Can you work these out from the model? Positions are in its coordinate system, mm. Face numbers are marked on the shaded views. A direction names the side the tool comes from. Round coordinates to 2 decimals unless told otherwise and drop trailing zeros. Loops run counter-clockwise (first coordinate to the right, second up) from the corner with the lowest first, then second, coordinate; pieces in that order, holes last. Notation, with made-up numbers: (7.25, 77.25) -> (55.25, 77.25) arc R35 ccw to (55.25, 116.25) -> close; hole circle Ø2 at (29, 16.5). An arc over 180 degrees is marked (long way). Write item = value, one per line.
from build123d import *

# Parameters (mm, degrees)
SKETCH1_W           = 86
SKETCH1_H           = 79
BOSS_EXTRUDE1_DEPTH = 36.5
CUT_EXTRUDE4_DEPTH  = 113.8543313
CUT_EXTRUDE6_DEPTH  = 117.39336237
SKETCH23_W          = 52.496433732
SKETCH23_H          = 95.180046085
CUT_EXTRUDE9_DEPTH  = 99.910462918
SKETCH26_W          = 80.038892534
SKETCH26_H          = 43.235962509
CUT_EXTRUDE10_DEPTH = 122.988754281
SKETCH27_R          = 10
BOSS_EXTRUDE2_DEPTH = 20
SKETCH28_R          = 9.1
CUT_EXTRUDE11_DEPTH = 20


with BuildPart() as part:
    # Sketch1 → Boss-Extrude1 (new body)
    with BuildSketch(Plane(origin=(0, 0, 0), x_dir=(1, 0, 0), z_dir=(0, 1, 0))):
        Polygon((-79.5, 16), (-79.5, -16), (-43, -39.5), (-43, 39.5), align=None)
        Rectangle(SKETCH1_W, SKETCH1_H)
    extrude(amount=BOSS_EXTRUDE1_DEPTH)

    # Sketch14 → Cut-Extrude4 (cut, through all)
    with BuildSketch(Plane(origin=(-24.252710924, -11.01949414, 37.669104201), x_dir=(0.8506873519118823, -0.14759139817848807, 0.5045273119275789), z_dir=(-0.5256719788015616, -0.23884502264638724, 0.8164692436705117))):
        Polygon((-9.224645292, 10.062781894), (-22.037813345, 46.122121953), (-64.94429352, 39.524095052), (-109.490464552, 32.673921521), (-56.610292459, -14.345266084), align=None)
    cut_extrude4 = extrude(amount=CUT_EXTRUDE4_DEPTH, mode=Mode.SUBTRACT)

    # Sketch15 → Cut-Extrude6 (cut, through all)
    with BuildSketch(Plane(origin=(0, -3.557773101, 35.48359566), x_dir=(1, 0, 0), z_dir=(0, -0.0997650710839227, 0.9950110203367698))):
        Polygon((43, 3.575611755), (43, 40.25862255), (-43, 40.25862255), (-38.621652742, -4.136841908), align=None)
    cut_extrude6 = extrude(amount=CUT_EXTRUDE6_DEPTH, mode=Mode.SUBTRACT)

    # Mirror7: Cut-Extrude4, Cut-Extrude6 across plane
    add(cut_extrude4.mirror(Plane.XY), mode=Mode.SUBTRACT)
    add(cut_extrude6.mirror(Plane.XY), mode=Mode.SUBTRACT)

    # Sketch23 → Cut-Extrude9 (cut, through all)
    with BuildSketch(Plane(origin=(-18.267826798, -30.352696834, 0), x_dir=(-0.8567921384922006, 0.515661935203639, 0), z_dir=(-0.515661935203639, -0.8567921384922006, 0))):
        with Locations((54.636530777, 2.381508201)):
            Rectangle(SKETCH23_W, SKETCH23_H)
    extrude(amount=CUT_EXTRUDE9_DEPTH, mode=Mode.SUBTRACT)

    # Sketch26 → Cut-Extrude10 (cut, through all)
    with BuildSketch(Plane(origin=(-35.634500138, -23.512575375, 31.888811139), x_dir=(0.4994950200350479, 0.3295798808101732, 0.8011752786533913), z_dir=(-0.6687218639205573, -0.4412401793127581, 0.598429756007053))):
        with Locations((-7.20146585, 56.642835767)):
            Rectangle(SKETCH26_W, SKETCH26_H)
    cut_extrude10 = extrude(amount=CUT_EXTRUDE10_DEPTH, mode=Mode.SUBTRACT)

    # Mirror9: Cut-Extrude10 across plane
    add(cut_extrude10.mirror(Plane.XY), mode=Mode.SUBTRACT)

    # Sketch27 → Boss-Extrude2 (add)
    with BuildSketch(Plane.ZY.offset(79.5)):
        with Locations((0, 23.5)):
            Circle(SKETCH27_R)
    extrude(amount=BOSS_EXTRUDE2_DEPTH)

    # Sketch28 → Cut-Extrude11 (cut)
    with BuildSketch(Plane.ZY.offset(99.5)):
        with Locations((0, 23.5)):
            Circle(SKETCH28_R)
    extrude(amount=-CUT_EXTRUDE11_DEPTH, mode=Mode.SUBTRACT)


solid = part.part
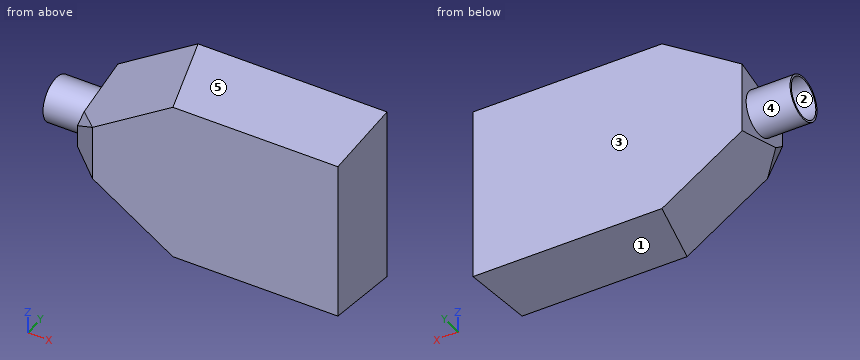
1. Suppose I cut it at C-C, the plane x = -27. List the corners of the cut face in (y, z) for me.
Entries:
outline = (0, -35.84) -> (36.5, -39.5) -> (36.5, 39.5) -> (0, 35.84) -> close
2. I need wall thicknesses on line 1 (Y direction, x = -90, z = 0); line 2 (Z direction, x = -88, y = 23); line 3 (X direction, y = 31.5, z = 13.5). Which ranges of each line are inside material? Lowest first, please. Write a range as [from, to].
Entries:
line_1 = [13.5, 14.4], [32.6, 33.5]
line_2 = [-9.99, -9.09], [9.09, 9.99]
line_3 = [-79.5, 43]
3. Suppose I cut it at B-B, the plane y = 4. List the corners of the cut face in (x, z) for me, and give its area (3 significant figures).
Entries:
outline = (-75.35, -7.8) -> (-72.46, -11.03) -> (-33.29, -36.24) -> (43, -36.24) -> (43, 36.24) -> (-33.29, 36.24) -> (-72.46, 11.03) -> (-75.35, 7.8) -> close
area = 7,440 mm²
4. For the marked faces 4 and 5, which set-ups out of +Z, -Z, +X, -X, +Y, -Y let a thin tool reach every point of the face, with its end or its side?
Entries:
face_4 = -X
face_5 = +Z, +X, -X, -Y
5. Suppose I cut it at A-A, the plane z = 0. List the corners of the cut face in (x, y) for me, and give its area (3 significant figures).
Entries:
outline = (-99.5, 13.5) -> (-79.5, 13.5) -> (-79.5, 6.5) -> (-68.7, 0) -> (43, 0) -> (43, 36.5) -> (-79.5, 36.5) -> (-79.5, 33.5) -> (-99.5, 33.5) -> (-99.5, 32.6) -> (-79.5, 32.6) -> (-79.5, 14.4) -> (-99.5, 14.4) -> close
area = 4,470 mm²
6. Suppose I cut it at D-D, the plane y = 23.5. List the corners of the cut face in (x, z) for me, and give its area (3 significant figures).
Entries:
outline = (-99.5, -10) -> (-79.5, -10) -> (-79.5, -12.2) -> (-39.12, -38.2) -> (43, -38.2) -> (43, 38.2) -> (-39.12, 38.2) -> (-79.5, 12.2) -> (-79.5, 10) -> (-99.5, 10) -> (-99.5, 9.1) -> (-79.5, 9.1) -> (-79.5, -9.1) -> (-99.5, -9.1) -> close
area = 8,340 mm²
7. We'd pull the mould along Y, two halves only. Please class the marked faces 1, 2 and 3: released by +Y, released by -Y, zero draft, split by the parting line, or undercut.
Entries:
face_1 = released by -Y
face_2 = undercut
face_3 = released by +Y
8. I'm going to push flat-ended pins straight in: pin 1 (2 mm diameter, centred on x = -80.5, y = 5, fed in from +Z); pin 2 (8 mm diameter, centred on y = 22.5, z = -27.5, fed in from -X); pin 3 (9 mm diameter, centred on y = 27.5, z = 4.5, fed in from -X); pin 4 (8 mm diameter, centred on x = -1.5, y = 4, fed in from +Z). Where does each tip first touch, or does it pass through?
Entries:
pin_1 = through
pin_2 = -61.75
pin_3 = -99.5
pin_4 = 36.64
